Source: CAD feature listing. Evaluate the final solid. Frame: model axes, mm. A direction names the side the tool comes from. Give positions to 0.01 mm unless a question says otherwise; leave off trailing zeros. Write each loop counter-clockwise with the first axis right and the second up, starting at its lowest first coordinate (ties: lowest second). Pieces come first, ordered by that corner, then holes. Notation, with made-up numbers: (-8, 20.25) -> (50, 20.25) arc R25 cw to (50, 55.25) -> close; hole circle Ø5 at (39, 25). An arc over 180 degrees is marked (long way). Use one line per item in the form item = value. Start each with the question number.
(1) First-contact query: P1, Ø1, axis at y = 135, z = 95.5, coming from the -X side; P2, Ø12, axis at x = 68, y = 105, coming from the +Z side. Flat tips, straight axial feed; report the tip coordinate or a pass-through.
(2) Cut plane A-A, the plane z = 119. Output: boundary loops of the cut face in (x, y), and give its area (3 significant figures).
(3) Material intervals for line 1 along X through (y, z) = (52, 95.5); line 2 along Z through (x, y) = (253, 122), sorted ascending. Write a range as from..to.
(4) Draft query along X for faces 3 (the face through (225, 79, 3)), 4 (the face through (231, 79, 0)), 5 (the face through (456, 79, 114)), 6 (the face through (0, 79, 111)). Return one class per face: pulls with the +X half, pulls with the -X half, needs draft (parallel to the pull), parting line crosses it, or undercut.
(5) Cut plane D-D, the plane z = 193.5. Output: boundary loops of the cut face in (x, y), and give its area (3 significant figures).
(6) Set-up query: faces 1 (the face through (1.521, 145.742, 209.964)), 2 (the face through (453, 79, 112)). Return all of +Z, -Z, +X, -X, +Y, -Y with unobstructed straight access to the full face (end or side cutting, diameter ignored); none if empty.
(7) Cut plane B-B, the plane y = 42. Output: boundary loops of the cut face in (x, z).
(8) Cut plane C-C, the plane x = 220.5. Output: boundary loops of the cut face in (y, z).
from build123d import *

# Parameters (mm, degrees)
SALIENTE_EXTRUIR1_DEPTH = 160
CORTAR_EXTRUIR1_DEPTH   = 456
CORTAR_EXTRUIR2_REACH   = 227
CROQUIS3_R              = 2.5
CROQUIS3_W              = 5
CROQUIS3_H              = 5
REDONDEO1_R             = 50


with BuildPart() as part:
    # Croquis1 → Saliente-Extruir1 (new body)
    with BuildSketch(Plane(origin=(0, 0, 0), x_dir=(1, 0, 0), z_dir=(0, 1, 0))):
        Polygon((3, -225), (3, -3), (453, -3), (453, -225), (456, -225), (456, 0), (0, 0), (0, -225), align=None)
    extrude(amount=SALIENTE_EXTRUIR1_DEPTH)

    # Croquis2 → Cortar-Extruir1 (cut)
    with BuildSketch(Plane.ZY):
        with BuildLine():
            ThreePointArc((65.5, 5), (63, 2.5), (60.5, 5))
            Line((60.5, 5), (60.5, 0))
            Line((60.5, 0), (65.5, 0))
            Line((65.5, 0), (65.5, 5))
        make_face()
        with BuildLine():
            ThreePointArc((65.5, 5), (63, 7.5), (60.5, 5))
            Line((60.5, 5), (65.5, 5))
        make_face()
        with BuildLine():
            Line((65.5, 5), (60.5, 5))
            ThreePointArc((60.5, 5), (63, 2.5), (65.5, 5))
        make_face()
        with BuildLine():
            ThreePointArc((135.5, 5), (133, 7.5), (130.5, 5))
            Line((130.5, 5), (135.5, 5))
        make_face()
        with BuildLine():
            Line((135.5, 5), (130.5, 5))
            ThreePointArc((130.5, 5), (133, 2.5), (135.5, 5))
        make_face()
        with BuildLine():
            Line((130.5, 5), (130.5, 0))
            Line((130.5, 0), (135.5, 0))
            Line((135.5, 0), (135.5, 5))
            ThreePointArc((135.5, 5), (133, 2.5), (130.5, 5))
        make_face()
    extrude(amount=-CORTAR_EXTRUIR1_DEPTH, mode=Mode.SUBTRACT)

    # Croquis3 → Cortar-Extruir2 (cut, up to next)
    with BuildSketch(Plane(origin=(0, 0, 0), x_dir=(-1, 0, 0), z_dir=(0, 0, -1)), mode=Mode.PRIVATE) as cortar_extruir2_sk1:
        with Locations((-348, 5)):
            Circle(CROQUIS3_R)
    cortar_extruir2_tool1 = extrude(cortar_extruir2_sk1.sketch, amount=-CORTAR_EXTRUIR2_REACH, mode=Mode.PRIVATE) & part.part
    add(cortar_extruir2_tool1.solids().sort_by_distance((348, 5, 0))[0], mode=Mode.SUBTRACT)
    # Croquis3 → Cortar-Extruir2 (cut, up to next)
    with BuildSketch(Plane(origin=(0, 0, 0), x_dir=(-1, 0, 0), z_dir=(0, 0, -1)), mode=Mode.PRIVATE) as cortar_extruir2_sk2:
        with Locations((-228, 5)):
            Circle(CROQUIS3_R)
    cortar_extruir2_tool2 = extrude(cortar_extruir2_sk2.sketch, amount=-CORTAR_EXTRUIR2_REACH, mode=Mode.PRIVATE) & part.part
    add(cortar_extruir2_tool2.solids().sort_by_distance((228, 5, 0))[0], mode=Mode.SUBTRACT)
    # Croquis3 → Cortar-Extruir2 (cut, up to next)
    with BuildSketch(Plane(origin=(0, 0, 0), x_dir=(-1, 0, 0), z_dir=(0, 0, -1)), mode=Mode.PRIVATE) as cortar_extruir2_sk3:
        with Locations((-108, 5)):
            Circle(CROQUIS3_R)
    cortar_extruir2_tool3 = extrude(cortar_extruir2_sk3.sketch, amount=-CORTAR_EXTRUIR2_REACH, mode=Mode.PRIVATE) & part.part
    add(cortar_extruir2_tool3.solids().sort_by_distance((108, 5, 0))[0], mode=Mode.SUBTRACT)
    # Croquis3 → Cortar-Extruir2 (cut, up to next)
    with BuildSketch(Plane(origin=(0, 0, 0), x_dir=(-1, 0, 0), z_dir=(0, 0, -1)), mode=Mode.PRIVATE) as cortar_extruir2_sk4:
        with Locations((-228, 2.5)):
            Rectangle(CROQUIS3_W, CROQUIS3_H)
    cortar_extruir2_tool4 = extrude(cortar_extruir2_sk4.sketch, amount=-CORTAR_EXTRUIR2_REACH, mode=Mode.PRIVATE) & part.part
    add(cortar_extruir2_tool4.solids().sort_by_distance((228, 2.5, 0))[0], mode=Mode.SUBTRACT)
    # Croquis3 → Cortar-Extruir2 (cut, up to next)
    with BuildSketch(Plane(origin=(0, 0, 0), x_dir=(-1, 0, 0), z_dir=(0, 0, -1)), mode=Mode.PRIVATE) as cortar_extruir2_sk5:
        with Locations((-108, 2.5)):
            Rectangle(CROQUIS3_W, CROQUIS3_H)
    cortar_extruir2_tool5 = extrude(cortar_extruir2_sk5.sketch, amount=-CORTAR_EXTRUIR2_REACH, mode=Mode.PRIVATE) & part.part
    add(cortar_extruir2_tool5.solids().sort_by_distance((108, 2.5, 0))[0], mode=Mode.SUBTRACT)
    # Croquis3 → Cortar-Extruir2 (cut, up to next)
    with BuildSketch(Plane(origin=(0, 0, 0), x_dir=(-1, 0, 0), z_dir=(0, 0, -1)), mode=Mode.PRIVATE) as cortar_extruir2_sk6:
        with Locations((-348, 2.5)):
            Rectangle(CROQUIS3_W, CROQUIS3_H)
    cortar_extruir2_tool6 = extrude(cortar_extruir2_sk6.sketch, amount=-CORTAR_EXTRUIR2_REACH, mode=Mode.PRIVATE) & part.part
    add(cortar_extruir2_tool6.solids().sort_by_distance((348, 2.5, 0))[0], mode=Mode.SUBTRACT)

    # Redondeo1
    redondeo1_edges = [part.edges().sort_by_distance(p)[0] for p in [
        (454.5, 160, 225),
        (1.5, 160, 225),
    ]]
    fillet(redondeo1_edges, radius=REDONDEO1_R)


solid = part.part
Geometry says:
q1.P1 = 0
q1.P2 = 3
q2.outline = (0, 0) -> (3, 0) -> (3, 160) -> (0, 160) -> close; (453, 0) -> (456, 0) -> (456, 160) -> (453, 160) -> close
q2.area = 960 mm^2
q3.line_1 = 0..3, 453..456
q3.line_2 = 0..3
q4.face_3 = undercut
q4.face_4 = needs draft
q4.face_5 = pulls with the +X half
q4.face_6 = pulls with the -X half
q5.outline = (0, 0) -> (3, 0) -> (3, 156.45) -> (0, 156.45) -> close; (453, 0) -> (456, 0) -> (456, 156.45) -> (453, 156.45) -> close
q5.area = 939 mm^2
q6.face_1 = +Z, +X, -X, +Y
q6.face_2 = +Z, +Y, -Y
q7.outline = (0, 0) -> (456, 0) -> (456, 225) -> (453, 225) -> (453, 3) -> (3, 3) -> (3, 225) -> (0, 225) -> close
q8.outline = (0, 0) -> (160, 0) -> (160, 3) -> (0, 3) -> close
